For this review, take the finished solid that the model builds, in its own axes (mm). Face numbers are marked on the shaded views. A direction names the side the tool comes from. Round coordinates to 2 decimals unless told otherwise and drop trailing zeros. Order: outer loops, then holes, each group sorted by start corner. A loop starts at its lowest first (then second) coordinate and runs counter-clockwise, first axis right, second up.
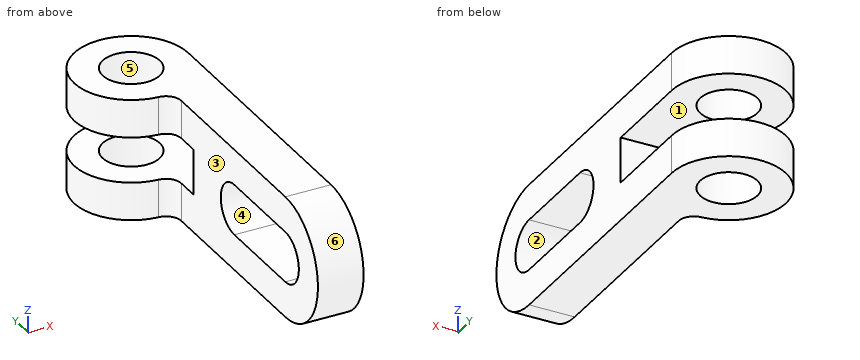
from build123d import *

# Parameters (mm, degrees)
F0_R     = 7.5
F1_DEPTH = 16
F3_W     = 10.303062
F3_H     = 12
F4_DEPTH = 12.001
F5_W     = 37.142856
F5_H     = 12
F6_DEPTH = 40.001
F7_R     = 4


with BuildPart() as f1:
    # F0 (on Top) → F1 (new body, symmetric)
    with BuildSketch(Plane.XY):
        with BuildLine():
            Line((15, -86.085342), (15, 0))
            ThreePointArc((15, 0), (-10.606602, 10.606602), (0, -15))
            ThreePointArc((0, -15), (1.507634, -14.924042), (3, -14.696938))
            Line((3, -14.696938), (3, -86.085342))
            Line((3, -86.085342), (15, -86.085342))
        make_face()
        Circle(F0_R, mode=Mode.SUBTRACT)
    extrude(amount=F1_DEPTH, both=True)

    # F3 (on face) → F4 (cut, through all)
    with BuildSketch(Plane(origin=(3, 0, 0), x_dir=(0, -1, 0), z_dir=(-1, 0, 0))):
        with BuildLine():
            ThreePointArc((70, 16), (86, 0), (70, -16))
            Line((70, -16), (86.085342, -16))
            Line((86.085342, -16), (86.085342, 16))
            Line((86.085342, 16), (70, 16))
        make_face()
        with BuildLine():
            ThreePointArc((45, 6.648935), (38.351065, 0), (45, -6.648935))
            Line((45, -6.648935), (70, -6.648935))
            ThreePointArc((70, -6.648935), (76.648935, 0), (70, 6.648935))
            Line((70, 6.648935), (45, 6.648935))
        make_face()
        with Locations((19.848469, 0)):
            Rectangle(F3_W, F3_H)
    extrude(amount=-F4_DEPTH, mode=Mode.SUBTRACT)

    # F5 (on offset) → F6 (cut, through all)
    with BuildSketch(Plane.YZ.offset(-25)):
        Rectangle(F5_W, F5_H)
    extrude(amount=F6_DEPTH, mode=Mode.SUBTRACT)

    # F7
    f7_edges = [f1.edges().sort_by_distance(p)[0] for p in [
        (3, -14.696938, -11),
        (3, -14.696938, 11),
    ]]
    fillet(f7_edges, radius=F7_R)


solid = f1.part
(1) Tool access review of the marked faces 1, 2 and 3: name each direction out of +Z, -Z, +X, -X, +Y, -Y from which nothing blocks a thin tool from reaching the whole face with its end or side.
(2) Draft analysis for pull direction Z (two halves, no side actions). For the marked faces 4, 5 and 6, state which applies: pulls with the +Z half, pulls with the -Z half, needs draft (parallel to the pull), parting line crosses it, or undercut.
(3) Add section A-A on y = -68. Give the boundary of the cut face in (x, z).
(4) Clearance check with flat-ended pins moving along their axes: P1, Ø4, axis at x = -3.5, z = -5.5, coming from the +Y side; P2, Ø2, axis at x = 10, z = -6.5, coming from the -Y side (3 decimals); P3, Ø9, axis at x = 0, y = 0, coming from the -Z side; P4, Ø4, axis at y = -37, z = 9.5, coming from the -X side. State where each tip first meets the part, or that it passes through.
(5) Add section C-C on z = 0. Give the boundary of the cut face in (x, y).
(6) Add section D-D on y = 4. Give the boundary of the cut face in (x, z), plus the area to 3 significant figures.
(7) Add section B-B on x = 6.5. Give the boundary of the cut face in (y, z), plus the area to 3 significant figures.
(8) Wall thickness on L1, parallel to X at y = 0, z = 10.75; L2, parallel to Z at x = -11, y = -5; L3, parallel to Z at x = 4.5, y = -50.5: over which ranges is each line inside the solid? List them lowest first.
Here are the results:
1. face 1: +X, -X, +Y
1. face 2: +X, -X
1. face 3: +Z, -Z, -X, -Y
2. face 4: undercut
2. face 5: needs draft
2. face 6: parting line crosses it
3. outline: (3, -16) - (15, -16) - (15, -6.65) - (3, -6.65) - close; (3, 6.65) - (15, 6.65) - (15, 16) - (3, 16) - close
4. P1: stops at y = 14.92
4. P2: stops at y = -85.025
4. P3: passes through
4. P4: stops at x = 3
5. outline: (3, -86) - (15, -86) - (15, -76.65) - (3, -76.65) - close; (3, -38.35) - (15, -38.35) - (15, -25) - (3, -25) - close
6. outline: (-14.46, -16) - (-6.34, -16) - (-6.34, -6) - (-14.46, -6) - close; (-14.46, 6) - (-6.34, 6) - (-6.34, 16) - (-14.46, 16) - close; (6.34, -16) - (14.46, -16) - (14.46, -6) - (6.34, -6) - close; (6.34, 6) - (14.46, 6) - (14.46, 16) - (6.34, 16) - close
6. area: 325 mm2
7. outline: (-70, -16) - (-3.74, -16) - (-3.74, -6) - (-25, -6) - (-25, 6) - (-3.74, 6) - (-3.74, 16) - (-70, 16) arc R16 ccw to start; (3.74, -16) - (13.52, -16) - (13.52, -6) - (3.74, -6) - close; (3.74, 6) - (13.52, 6) - (13.52, 16) - (3.74, 16) - close; hole (-70, -6.65) - (-45, -6.65) arc R6.65 ccw to (-45, 6.65) - (-70, 6.65) arc R6.65 ccw to start
7. area: 1,990 mm2
8. L1: x = -15 to -7.5, 7.5 to 15
8. L2: z = -16 to -6, 6 to 16
8. L3: z = -16 to -6.65, 6.65 to 16
